from build123d import *

# Parameters (mm, degrees)
SKETCH_1_R      = 2.1
EXTRUDE_1_DEPTH = 6


with BuildPart() as part:
    # 스케치1 → 보스-돌출1 (new, symmetric)
    with BuildSketch(Plane(origin=(0, 0, 0), x_dir=(0, 0, -1), z_dir=(1, 0, 0))):
        with BuildLine():
            Line((-16.843616133, 15.225059748), (-5.058260457, 18.301873078))
            Line((-5.058260457, 18.301873078), (-3.370048504, 17.287466348))
            Line((-3.370048504, 17.287466348), (-4.598836935, 12.46676509))
            Line((-4.598836935, 12.46676509), (0.718846359, 11.548294979))
            Line((0.718846359, 11.548294979), (1.44805016, 16.220144947))
            Line((1.44805016, 16.220144947), (9.090162136, 14.827237538))
            Line((9.090162136, 14.827237538), (18.490753638, -3.782754553))
            Line((18.490753638, -3.782754553), (16.165658803, -8.432944223))
            Line((16.165658803, -8.432944223), (7.383267841, -5.77780277))
            Line((7.383267841, -5.77780277), (8.431827356, -21.818977094))
            Line((8.431827356, -21.818977094), (1.737192047, -20.750684226))
            Line((1.737192047, -20.750684226), (-0.33854919, -10.977402568))
            Line((-0.33854919, -10.977402568), (-4.598836935, -10.297569417))
            Line((-4.598836935, -10.297569417), (-5.563105297, -2.251013026))
            Line((-5.563105297, -2.251013026), (-15.432595358, 7.537806593))
            Line((-15.432595358, 7.537806593), (-16.755575012, 7.849664338))
            ThreePointArc((-16.755575012, 7.849664338), (-19.683449159, 11.502937082), (-16.843616133, 15.225059748))
        make_face()
        Circle(SKETCH_1_R, mode=Mode.SUBTRACT)
    extrude(amount=EXTRUDE_1_DEPTH, both=True)


solid = part.part
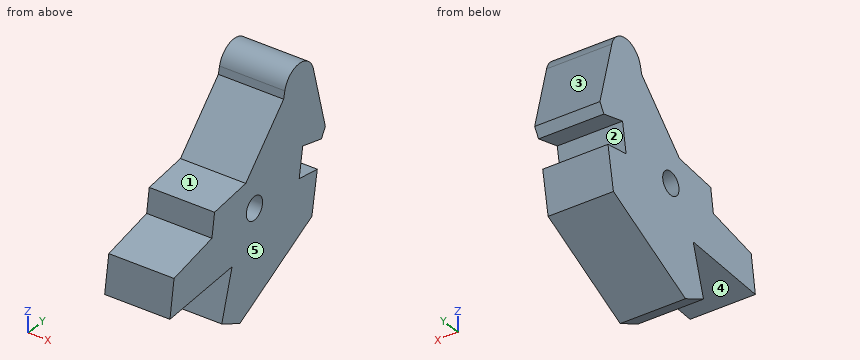
Design review of the part built by this model. Coordinates are the model's own, in mm. Face numbers are marked on the shaded views. A direction names the side the tool comes from. Coordinates: 2 decimals unless noted, no trailing zeros. Order: outer loops, then holes, each group sorted by start corner. A loop starts at its lowest first (then second) coordinate and runs counter-clockwise, first axis right, second up. Notation, with made-up numbers: (23, 57.5) - (70, 57.5) arc R29 ccw to (70, 95.5) - close; hole circle Ø3 at (67.5, -23.5). An arc over 180 degrees is marked (long way). Put each result on its own line as item: value.
1) Take a section at C-C, the plane y = -14. Give the boundary of the cut face in (x, z), and give its area (3 significant figures).
Response values:
outline: (-6, -7.92) - (6, -7.92) - (6, -0.3) - (-6, -0.3) - close
area: 91.4 mm²
2) Take a section at B-B, the plane y = 0. Give the boundary of the cut face in (x, z).
Response values:
outline: (-6, -16.58) - (6, -16.58) - (6, -2.1) - (-6, -2.1) - close; (-6, 2.1) - (6, 2.1) - (6, 7.83) - (-6, 7.83) - close
3) Wall thickness on L1, parallel to Z at x = -4.5, y = 13; L2, parallel to Z at x = 5, y = -8.5; L3, parallel to Y at x = 0.25, z = 14: over which ranges is each line inside the solid? List them lowest first. Write a range as from..to.
Response values:
L1: z = -10.01..-0.95, 4.46..19.4
L2: z = -7.56..4.81
L3: y = 6.12..15.97
4) Insertion check: P1, Ø1, axis at x = 2, y = -4.5, coming from the -Z side; P2, Ø3, axis at x = -1.5, z = 2, coming from the +Y side; P3, Ø5, axis at x = -2, y = 7, coming from the +Z side; P4, Ø3.5, axis at y = 0, z = 0, coming from the +X side. Each pin has a flat end and moves straight along its axis. Give the tip position at first contact, or say it passes through.
Response values:
P1: stops at z = -18.38
P2: stops at y = 17.37
P3: stops at z = 19.08
P4: passes through
5) Take a section at A-A, the plane x = 1.5. Give the boundary of the cut face in (y, z).
Response values:
outline: (-21.82, -8.43) - (-5.78, -7.38) - (-8.43, -16.17) - (-3.78, -18.49) - (14.83, -9.09) - (16.22, -1.45) - (11.55, -0.72) - (12.47, 4.6) - (17.29, 3.37) - (18.3, 5.06) - (15.23, 16.84) arc R3.8 ccw to (7.85, 16.76) - (7.54, 15.43) - (-2.25, 5.56) - (-10.3, 4.6) - (-10.98, 0.34) - (-20.75, -1.74) - close; hole circle Ø4.2 at (0, 0)
6) Take a section at D-D, the plane z = 9. Give the boundary of the cut face in (x, y), and give its area (3 significant figures).
Response values:
outline: (-6, 1.16) - (6, 1.16) - (6, 17.27) - (-6, 17.27) - close
area: 193 mm²
7) Tool access review of the marked faces 1 and 2: name each direction out of +Z, -Z, +X, -X, +Y, -Y from which nothing blocks a thin tool from reaching the whole face with its end or side.
Response values:
face 1: +Z, +X, -X, -Y
face 2: +X, -X
8) The part is to be moulded in two halves that separate along Y. For the marked faces 3, 4 and 5, say which applies: released by +Y, released by -Y, zero draft, split by the parting line, or undercut.
Response values:
face 3: released by +Y
face 4: undercut
face 5: zero draft
